Check sheet for the modelled part. Datum: model origin and axes. Units: mm. A direction names the side the tool comes from. Round coordinates to 2 decimals unless told otherwise and drop trailing zeros. Write each loop counter-clockwise with the first axis right and the second up, starting at its lowest first coordinate (ties: lowest second). Pieces come first, ordered by that corner, then holes. Notation, with made-up numbers: (71.5, 37.5) - (83.5, 37.5) arc R22 cw to (83.5, 59.5) - close; hole circle Ø5 at (39.25, -31). An arc over 180 degrees is marked (long way). Answer as a JSON object with one key per item and string values. Group by question number.
Item 1: Release check for a two-part mould opening along X. For faces 1 (the flat face through (0.07, -1.779, 3.756)), 2 (the flat face through (5, -1, 0)), 3 (the cylindrical face through (1.64, -1.28, 1.26)) record: pulls with the +X half, pulls with the -X half, needs draft (parallel to the pull), parting line crosses it, or undercut.
Item 2: Gauge pin test, flat ends, axial feed: P1, Ø1.5, axis at x = -3.5, y = 0.5, coming from the -Z side; P2, Ø2, axis at x = 2, z = 4, coming from the +Y side; P3, Ø1.5, axis at x = 1.5, z = -3.5, coming from the +Y side; P4, Ø0.7, axis at x = 0, y = 0.5, coming from the -Z side. Record the tip position at first contact, or that the pin passes through.
Item 3: Sectioned sample at A-A on z = 1.75. Record the boundary of the cut face in (x, y), plus the area to 3 significant figures.
Item 4: Thickness scan on line 1 (X direction, y = -0.1, z = -0.75); line 2 (Z direction, x = 0, y = -0.8); line 3 (Z direction, x = 0, y = -2). Record the ranges inside material, lowest first.
Item 5: Sectioned sample at C-C on y = -1.3. Record the boundary of the cut face in (x, z), plus the area to 3 significant figures.
Item 6: Set-up check for faces 4 (the flat face through (-5, -1, 0)), 5 (the flat face through (0, 0, -4)), 6 (the flat face through (0, 0, 4)): record each of +Z, -Z, +X, -X, +Y, -Y from which the full face is reachable in a straight line by a thin tool's end or side.
Item 7: Sectioned sample at B-B on x = 0. Record the boundary of the cut face in (y, z).
Item 8: Sectioned sample at D-D on x = -3.5. Record the boundary of the cut face in (y, z).
```python
from build123d import *

# Parameters (mm, degrees)
BOSS_EXTRUDE1_DEPTH = 5
FILLET1_R           = 0.3
FILLET2_R           = 0.2
TAPPED_HOLE1_D      = 4.134


with BuildPart() as part:
    # Sketch1 → Boss-Extrude1 (new, symmetric)
    with BuildSketch(Plane(origin=(0, 0, 0), x_dir=(0, 0, -1), z_dir=(1, 0, 0))):
        with BuildLine():
            Line((2.5, -3.3), (-2.5, -3.3))
            Line((-2.5, -3.3), (-4.954229367, -0.327331466))
            ThreePointArc((-4.954229367, -0.327331466), (-4.980923041, -0.114754159), (-4.8, 0))
            Line((-4.8, 0), (-2.9, 0))
            Line((-2.9, 0), (-2.9, 0.8))
            Line((-2.9, 0.8), (2.9, 0.8))
            Line((2.9, 0.8), (2.9, 0))
            Line((2.9, 0), (4.8, 0))
            ThreePointArc((4.8, 0), (4.980923041, -0.114754159), (4.954229367, -0.327331466))
            Line((4.954229367, -0.327331466), (2.5, -3.3))
        make_face()
    extrude(amount=BOSS_EXTRUDE1_DEPTH, both=True)

    # Fillet1
    fillet1_edges = [part.edges().sort_by_distance(p)[0] for p in [
        (0, -3.3, -2.5),
        (0, -3.3, 2.5),
    ]]
    fillet(fillet1_edges, radius=FILLET1_R)

    # Fillet2
    fillet2_edges = [part.edges().sort_by_distance(p)[0] for p in [
        (0, 0.8, 2.9),
        (0, 0.8, -2.9),
    ]]
    fillet(fillet2_edges, radius=FILLET2_R)

    # Tapped Hole1 (through all)
    with Locations(Plane(origin=(0, 0.8, 0), x_dir=(1, 0, 0), z_dir=(0, 1, 0))):
        with Locations((0, 0)):
            Hole(TAPPED_HOLE1_D / 2)


solid = part.part
```
Completed:
{
 "1": {"face 1": "needs draft", "face 2": "pulls with the +X half", "face 3": "undercut"},
 "2": {"P1": "z = -5", "P2": "y = 0", "P3": "y = 0.79", "P4": "z = -2.9"},
 "3": {"outline": "(-5, -3.3) - (-1.1, -3.3) - (-1.1, 0.8) - (-5, 0.8) - close; (1.1, -3.3) - (5, -3.3) - (5, 0.8) - (1.1, 0.8) - close", "area": "32.0 mm²"},
 "4": {"line 1": "-5 to -1.93, 1.93 to 5", "line 2": "-4.56 to -2.07, 2.07 to 4.56", "line 3": "-3.57 to -2.07, 2.07 to 3.57"},
 "5": {"outline": "(-5, -4.15) - (5, -4.15) - (5, 4.15) - (-5, 4.15) - close; hole circle Ø4.13 at (0, 0)", "area": "69.6 mm²"},
 "6": {"face 4": "+Z, -Z, -X, +Y, -Y", "face 5": "-Z, +X, -X, +Y", "face 6": "+Z, +X, -X, +Y"},
 "7": {"outline": "(-3.3, -2.36) arc R0.3 ccw to (-3.19, -2.59) - (-0.33, -4.95) arc R0.2 ccw to (0, -4.8) - (0, -2.9) - (0.6, -2.9) arc R0.2 ccw to (0.8, -2.7) - (0.8, -2.07) - (-3.3, -2.07) - close; (-3.3, 2.07) - (0.8, 2.07) - (0.8, 2.7) arc R0.2 ccw to (0.6, 2.9) - (0, 2.9) - (0, 4.8) arc R0.2 ccw to (-0.33, 4.95) - (-3.19, 2.59) arc R0.3 ccw to (-3.3, 2.36) - close"},
 "8": {"outline": "(-3.3, -2.36) arc R0.3 ccw to (-3.19, -2.59) - (-0.33, -4.95) arc R0.2 ccw to (0, -4.8) - (0, -2.9) - (0.6, -2.9) arc R0.2 ccw to (0.8, -2.7) - (0.8, 2.7) arc R0.2 ccw to (0.6, 2.9) - (0, 2.9) - (0, 4.8) arc R0.2 ccw to (-0.33, 4.95) - (-3.19, 2.59) arc R0.3 ccw to (-3.3, 2.36) - close"}
}
